Read the model definition and answer for the solid it produces. Units are mm, in the model's axes. A direction names the side the tool comes from. Round coordinates to 2 decimals unless told otherwise and drop trailing zeros. Order: outer loops, then holes, each group sorted by start corner. A loop starts at its lowest first (then second) coordinate and runs counter-clockwise, first axis right, second up. Notation, with made-up numbers: M -21.5,86.5 L 11.5,86.5 A16 cw 11.5,111.5 Z; hole C -4,51.5 d11. An arc over 180 degrees is marked long. Answer as CSV lines item,"result".
```python
from build123d import *


with BuildPart() as part:
    # Esquisse1 → Révolution1 (revolve)
    with BuildSketch(Plane.XY):
        Polygon((0, 0), (0, 3.5), (-25, 3.5), (-26.5, 5), (-35, 5), (-35, 4.25), (-36.5, 4.25), (-36.5, 5), (-49, 5), (-50, 4), (-50, 0), align=None)
    r_volution1 = revolve(axis=Axis((-50, 0, 0), (1, 0, 0)))

    # Symétrie1: Révolution1 across Right Plane
    add(r_volution1.mirror(Plane(origin=(0, 0, 0), x_dir=(0, 0, -1), z_dir=(1, 0, 0))))


solid = part.part
```
Item 1: A cutting plane is placed at D-D, the plane x = 10.5. Determine the outline of the cut face in (y, z).
Ans:
outline,"C 0,0 d7"
Item 2: Flat-ended cylindrical pins translate along their axes: pin 1 (2 mm diameter, centred on x = 1, z = 3.5, fed in from -Y); pin 2 (1.5 mm diameter, centred on x = -18.5, z = -1, fed in from -Y); pin 3 (5 mm diameter, centred on x = 39.5, z = -3, fed in from -Y). Find the tip coordinate at first contact, or state that the pin passes through.
Ans:
pin 1,"y = -2.45"
pin 2,"y = -3.49"
pin 3,"y = -4.97"
Item 3: Determine the mould class of faces 1 (the face through (-50, 0, 0)), 2 (the face through (50, 0, 0)), 3 (the face through (-42.84, -1.08, -4.88)), 4 (the face through (-35, -2, -4)) for opening direction X: +X half, -X half, draft (parallel to the pull), parting line (faces both ways), or undercut.
Ans:
face 1,"-X half"
face 2,"+X half"
face 3,"draft"
face 4,"undercut"
Item 4: A cutting plane is placed at C-C, the plane x = 27.5. Determine the outline of the cut face in (y, z).
Ans:
outline,"C 0,0 d10"
Item 5: A tool of negligible diameter and unlimited length cuts with its end or side. For faces 5 (the face through (42.84, -1.08, -4.88)), 6 (the face through (35.76, 2.285, 3.584)), from which of +Z, -Z, +X, -X, +Y, -Y can it reach the whole face along a straight path? Write none if from no direction.
Ans:
face 5,"+X, -X"
face 6,"none"
Item 6: Find the intervals of material crossed by probe 1 along X at (y, z) = (3.75, -3.25); probe 2 along X at (y, z) = (4.25, -2.25); probe 3 along Z at (x, y) = (-14, -0.25), in increasing order. Write a range as [from, to].
Ans:
probe 1,"[-49.04, -36.5], [-35, -26.46], [26.46, 35], [36.5, 49.04]"
probe 2,"[-49.19, -36.5], [-35, -26.31], [26.31, 35], [36.5, 49.19]"
probe 3,"[-3.49, 3.49]"
